Check sheet for the modelled part. Datum: model origin and axes. Units: mm. Round coordinates to 2 decimals unless told otherwise and drop trailing zeros. Write each loop counter-clockwise with the first axis right and the second up, starting at its lowest first coordinate (ties: lowest second). Pieces come first, ordered by that corner, then holes.
Item 1: Material ranges on line 1 (Y direction, x = 32.5, z = 0.4); line 2 (X direction, y = -13.5, z = 1.7); line 3 (Y direction, x = -32.3, z = 0.8), recorded low to high.
Item 2: Go/stop test with flat-tipped pins: pin 1 Ø1 at (x, z) = (-3, 2) entering from -Y; pin 2 Ø1.5 at (x, y) = (-14, 11) entering from -Z; pin 3 Ø2 at (x, y) = (-32.3, -22.5) entering from +Z. Record where each tip stops, or that it passes through.
Item 3: Cross-section at A-A on y = -1. Enter the section's corners in (x, z), plus the area to 3 significant figures.
Item 4: Cross-section at B-B on x = 21. Enter the section's corners in (y, z).
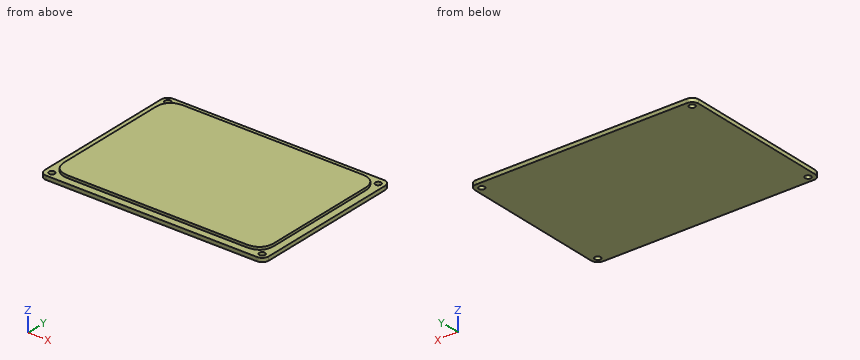
from build123d import *

# Parameters (mm, degrees)
F0_W        = 64.6
F0_H        = 44.6
F1_DEPTH    = 2
F0_W_2      = 69
F0_H_2      = 49
F2_DEPTH    = 1.2
F3_T1_DEPTH = 13.3
F4_R        = 2
F6_D        = 1.8
F6_DEPTH    = 6
F6_TIP      = 0.5407745571


# Not quite as in the source:
# - a fillet or chamfer that OpenCascade refuses, or shapes differently, is made with other operations: its cross-section is extruded or revolved along the edge and cut away or added
# - the program builds the solid bodies; features that only make, move or delete a surface that nothing else refers to are left out


with BuildPart() as f1:
    # F0 (on Top) → F1 (new body)
    with BuildSketch(Plane.XY):
        Rectangle(F0_W, F0_H)
    extrude(amount=F1_DEPTH)

    # F0 (on Top) → F2 (join)
    with BuildSketch(Plane.XY):
        Rectangle(F0_W_2, F0_H_2)
        Rectangle(F0_W, F0_H, mode=Mode.SUBTRACT)
    extrude(amount=F2_DEPTH)

    # F3: fillet of radius 5 on 4 edges, made by hand

    # F3_s2 → F3_t1 (cut)
    with BuildSketch(Plane.XY.offset(1.2)):
        with BuildLine():
            add(Edge.make_bspline(
                [(-32.3, -17.3), (-32.3, -22.3), (-27.3, -22.3)],
                knots=[0, 0, 0, 1, 1, 1], degree=2, weights=[1, 1, 1]))
            Line((-27.3, -22.3), (-32.3, -22.3))
            Line((-32.3, -22.3), (-32.3, -17.3))
        make_face()
        with BuildLine():
            add(Edge.make_bspline(
                [(32.3, -17.3), (32.3, -22.3), (27.3, -22.3)],
                knots=[0, 0, 0, 1, 1, 1], degree=2, weights=[1, 1, 1]))
            Line((27.3, -22.3), (32.3, -22.3))
            Line((32.3, -22.3), (32.3, -17.3))
        make_face()
        with BuildLine():
            add(Edge.make_bspline(
                [(27.3, 22.3), (32.3, 22.3), (32.3, 17.3)],
                knots=[0, 0, 0, 1, 1, 1], degree=2, weights=[1, 1, 1]))
            Line((32.3, 17.3), (32.3, 22.3))
            Line((32.3, 22.3), (27.3, 22.3))
        make_face()
        with BuildLine():
            add(Edge.make_bspline(
                [(-27.3, 22.3), (-32.3, 22.3), (-32.3, 17.3)],
                knots=[0, 0, 0, 1, 1, 1], degree=2, weights=[1, 1, 1]))
            Line((-32.3, 17.3), (-32.3, 22.3))
            Line((-32.3, 22.3), (-27.3, 22.3))
        make_face()
    extrude(amount=F3_T1_DEPTH, mode=Mode.SUBTRACT)

    # F4
    f4_edges = [f1.edges().sort_by_distance(p)[0] for p in [
        (-34.5, 24.5, 0.6),
        (-34.5, -24.5, 0.6),
        (34.5, 24.5, 0.6),
        (34.5, -24.5, 0.6),
    ]]
    fillet(f4_edges, radius=F4_R)

    # F6
    with Locations(Plane.XY.offset(1.2)):
        with Locations((-32.3, -22.5), (-32.5, 22.5), (32.5, -22.5), (32.5, 22.3)):
            Hole(F6_D / 2, depth=F6_DEPTH)
            with Locations((0, 0, -(F6_DEPTH + F6_TIP / 2))):  # 118° drill point
                Cone(0, F6_D / 2, F6_TIP, mode=Mode.SUBTRACT)


solid = f1.part
Response values:
1. line 1: y = -24.5 to -23.4, -21.6 to 21.4, 23.2 to 24.5
1. line 2: x = -32.3 to 32.3
1. line 3: y = -24.5 to -23.4, -21.6 to 21.62, 23.38 to 24.5
2. pin 1: stops at y = -22.3
2. pin 2: stops at z = 0
2. pin 3: stops at z = 1.2
3. outline: (-34.5, 0) - (34.5, 0) - (34.5, 1.2) - (32.3, 1.2) - (32.3, 2) - (-32.3, 2) - (-32.3, 1.2) - (-34.5, 1.2) - close
3. area: 134 mm2
4. outline: (-24.5, 0) - (24.5, 0) - (24.5, 1.2) - (22.3, 1.2) - (22.3, 2) - (-22.3, 2) - (-22.3, 1.2) - (-24.5, 1.2) - close
